Autodesk Inventor part; units mm, degrees
ref_plane "YZ Plane" through (0, 0, 0) normal (1, 0, 0) x (0, 1, 0)
ref_plane "XZ Plane" through (0, 0, 0) normal (0, 1, 0) x (-1, 0, 0)
ref_plane "XY Plane" through (0, 0, 0) normal (0, 0, 1) x (1, 0, 0)
sketch "Эскиз1" plane through (0, 0, 0) normal (0, 1, 0) x (-1, 0, 0)
  line L0 (75.318, 42.5) -> (-75.318, 42.5)
  line L1 (-75.318, 42.5) -> (-75.318, -42.5)
  line L2 (-75.318, -42.5) -> (75.318, -42.5)
  line L3 (75.318, -42.5) -> (75.318, 42.5)
  line L4 (75.318, 42.5) -> (-75.318, -42.5) construction
  line L5 (-75.318, 42.5) -> (75.318, -42.5) construction
  point P0 (0, 0)
  dimension "d0" = 150.636
  dimension "d1" = 85
extrude "Выдавливание1" add sketch "Эскиз1" along normal mid plane 3
sketch "Эскиз3" plane through (-75.318, -1.5, 42.5) normal (-1, 0, 0) x (0, 0, 1)
  line L0 (-85, 0) -> (0, 0)
  line L1 (-80, 3) -> (-70, 3)
  line L2 (-70, 3) -> (-70, 0)
  line L3 (-70, 0) -> (-80, 0)
  line L4 (-80, 0) -> (-80, 3)
  line L5 (-80, 3) -> (-70, 0) construction
  line L6 (-70, 3) -> (-80, 0) construction
  line L7 (-60, 3) -> (-50, 3)
  line L8 (-50, 3) -> (-50, 0)
  line L9 (-50, 0) -> (-60, 0)
  line L10 (-60, 0) -> (-60, 3)
  line L11 (-60, 3) -> (-50, 0) construction
  line L12 (-50, 3) -> (-60, 0) construction
  line L13 (-35, 3) -> (-25, 3)
  line L14 (-25, 3) -> (-25, 0)
  line L15 (-25, 0) -> (-35, 0)
  line L16 (-35, 0) -> (-35, 3)
  line L17 (-35, 3) -> (-25, 0) construction
  line L18 (-25, 3) -> (-35, 0) construction
  line L19 (-15, 3) -> (-5, 3)
  line L20 (-5, 3) -> (-5, 0)
  line L21 (-5, 0) -> (-15, 0)
  line L22 (-15, 0) -> (-15, 3)
  line L23 (-15, 3) -> (-5, 0) construction
  line L24 (-5, 3) -> (-15, 0) construction
  line L25 (0, 0) -> (0, 3)
  line L26 (-85, 0) -> (-85, 3)
  point P0 (-42.5, 1.5)
  point P1 (-75, 1.5)
  point P2 (-55, 1.5)
  point P3 (-30, 1.5)
  point P4 (-10, 1.5)
  point P5 (-15, 1.5)
  point P6 (-25, 1.5)
  point P7 (-60, 1.5)
  point P8 (-35, 0)
  point P9 (-15, 0)
  dimension "d8" = 10
  dimension "d9" = 10
  dimension "d10" = 10
  dimension "d11" = 10
  dimension "d12" = 3
  dimension "d13" = 10
  dimension "d14" = 10
  dimension "d15" = 5
  dimension "d16" = 5
extrude "Выдавливание3" add sketch "Эскиз3" along normal blind 3
sketch "Эскиз4" plane through (75.318, -1.5, -42.5) normal (1, 0, 0) x (0, 0, -1)
  line L0 (-85, 3) -> (0, 3)
  line L1 (-80, 0.0026) -> (-70, 0.0026)
  line L2 (-70, 0.0026) -> (-70, 3)
  line L3 (-70, 3) -> (-80, 3)
  line L4 (-80, 3) -> (-80, 0.0026)
  line L5 (-80, 0.0026) -> (-70, 3) construction
  line L6 (-70, 0.0026) -> (-80, 3) construction
  line L7 (-60, 0.0026) -> (-50, 0.0026)
  line L8 (-50, 0.0026) -> (-50, 3)
  line L9 (-50, 3) -> (-60, 3)
  line L10 (-60, 3) -> (-60, 0.0026)
  line L11 (-60, 0.0026) -> (-50, 3) construction
  line L12 (-50, 0.0026) -> (-60, 3) construction
  line L13 (-42.5, 3) -> (-42.5, 0) construction
  line L14 (0, 0) -> (-85, 0)
  line L15 (-5, 0.0026) -> (-15, 0.0026)
  line L16 (-15, 0.0026) -> (-15, 3)
  line L17 (-15, 3) -> (-5, 3)
  line L18 (-5, 3) -> (-5, 0.0026)
  line L19 (-5, 0.0026) -> (-15, 3) construction
  line L20 (-15, 0.0026) -> (-5, 3) construction
  line L21 (-25, 0.0026) -> (-35, 0.0026)
  line L22 (-35, 0.0026) -> (-35, 3)
  line L23 (-35, 3) -> (-25, 3)
  line L24 (-25, 3) -> (-25, 0.0026)
  line L25 (-25, 0.0026) -> (-35, 3) construction
  line L26 (-35, 0.0026) -> (-25, 3) construction
  line L27 (-85, 3) -> (-85, 0)
  point P0 (-42.5, 1.5)
  point P1 (-75, 1.5013)
  point P2 (-55, 1.5013)
  point P3 (-10, 1.5013)
  point P4 (-30, 1.5013)
  point P5 (-35, 3)
  point P6 (-5, 3)
  point P7 (-15, 3)
  dimension "d19" = 10
  dimension "d24" = 20
  dimension "d29" = 5
extrude "Выдавливание4" add sketch "Эскиз4" along normal blind 3
sketch "Эскиз5" plane through (0, 1.5, 0) normal (0, 1, 0) x (1, 0, 0)
  line L0 (-75.318, 7.5) -> (-75.318, -7.5)
  line L1 (-54.4999, -2.8628) -> (-54.4999, -9.8628)
  line L2 (-54.4999, -9.8628) -> (-48.4999, -9.8628)
  line L3 (-48.4999, -9.8628) -> (-48.4999, -2.8628)
  line L4 (-48.4999, -2.8628) -> (-54.4999, -2.8628)
  line L5 (-48.4999, 3.1372) -> (-48.4999, 10.1372)
  line L6 (-48.4999, 10.1372) -> (-54.4999, 10.1372)
  line L7 (-54.4999, 10.1372) -> (-54.4999, 3.1372)
  line L8 (-54.4999, 3.1372) -> (-48.4999, 3.1372)
  line L9 (-51.4999, -2.8628) -> (-51.4999, 3.1372)
  circle A0 centre (-51.4999, 0.1372) radius 1.5
  point P0 (0, 0)
  dimension "d37" = 3
extrude "Выдавливание5" cut sketch "Эскиз5" against normal blind 3
sketch "Эскиз6" plane through (0, 1.5, 0) normal (0, 1, 0) x (1, 0, 0)
  line L0 (75.318, -27.5) -> (75.318, -17.5)
  line L1 (60.318, -24) -> (60.318, -21)
  line L2 (75.318, -21) -> (75.318, -24)
  line L3 (67.818, -25.55) -> (65.318, -25.55)
  line L4 (65.318, -19.45) -> (67.818, -19.45)
  line L5 (67.818, -19.45) -> (67.818, -21)
  line L6 (67.818, -24) -> (67.818, -25.55)
  line L7 (75.318, -24) -> (67.818, -24)
  line L8 (65.318, -24) -> (60.318, -24)
  line L9 (65.318, -25.55) -> (65.318, -24)
  line L10 (65.318, -21) -> (65.318, -19.45)
  line L11 (60.318, -21) -> (65.318, -21)
  line L12 (67.818, -21) -> (75.318, -21)
  line L13 (66.568, 0) -> (53.2147, 0) construction
  line L14 (0, -10.2584) -> (0, 8.5624) construction
  line L15 (75.318, 27.5) -> (75.318, 17.5)
  line L16 (60.318, 24) -> (60.318, 21)
  line L17 (75.318, 21) -> (75.318, 24)
  line L18 (67.818, 25.55) -> (65.318, 25.55)
  line L19 (65.318, 19.45) -> (67.818, 19.45)
  line L20 (67.818, 19.45) -> (67.818, 21)
  line L21 (67.818, 24) -> (67.818, 25.55)
  line L22 (75.318, 24) -> (67.818, 24)
  line L23 (65.318, 24) -> (60.318, 24)
  line L24 (65.318, 25.55) -> (65.318, 24)
  line L25 (65.318, 21) -> (65.318, 19.45)
  line L26 (60.318, 21) -> (65.318, 21)
  line L27 (67.818, 21) -> (75.318, 21)
  line L28 (0, 10.2584) -> (0, -8.5624) construction
  line L29 (-75.318, -27.5) -> (-75.318, -17.5)
  line L30 (-60.318, -24) -> (-60.318, -21)
  line L31 (-75.318, -21) -> (-75.318, -24)
  line L32 (-67.818, -25.55) -> (-65.318, -25.55)
  line L33 (-65.318, -19.45) -> (-67.818, -19.45)
  line L34 (-67.818, -19.45) -> (-67.818, -21)
  line L35 (-67.818, -24) -> (-67.818, -25.55)
  line L36 (-75.318, -24) -> (-67.818, -24)
  line L37 (-65.318, -24) -> (-60.318, -24)
  line L38 (-65.318, -25.55) -> (-65.318, -24)
  line L39 (-65.318, -21) -> (-65.318, -19.45)
  line L40 (-60.318, -21) -> (-65.318, -21)
  line L41 (-67.818, -21) -> (-75.318, -21)
  line L42 (-66.568, 0) -> (-53.2147, 0) construction
  line L43 (-60.318, 24) -> (-60.318, 21)
  line L44 (-65.318, 24) -> (-60.318, 24)
  line L45 (-60.318, 21) -> (-65.318, 21)
  line L46 (-65.318, 21) -> (-65.318, 19.45)
  line L47 (-65.318, 19.45) -> (-67.818, 19.45)
  line L48 (-67.818, 19.45) -> (-67.818, 21)
  line L49 (-65.318, 25.55) -> (-65.318, 24)
  line L50 (-67.818, 25.55) -> (-65.318, 25.55)
  line L51 (-67.818, 24) -> (-67.818, 25.55)
  line L52 (-67.818, 21) -> (-75.318, 21)
  line L53 (-75.318, 21) -> (-75.318, 24)
  line L54 (-75.318, 27.5) -> (-75.318, 17.5)
  line L55 (-75.318, 24) -> (-67.818, 24)
  point P0 (0, 0)
  point P1 (67.818, -23.3834)
  point P2 (67.818, 23.3834)
  point P3 (-67.818, -23.3834)
  point P4 (-67.818, 23.3834)
  point P5 (-75.318, -21)
  point P6 (75.318, -22.5)
  dimension "d38" = 6.1
  dimension "d39" = 3
  dimension "d40" = 2.5
  dimension "d41" = 15
  dimension "d42" = 1.55
  dimension "d43" = 1.55
  dimension "d44" = 1.55
  dimension "d45" = 1.55
extrude "Выдавливание6" cut sketch "Эскиз6" against normal blind 3
properties part number "Нижняя часть головы"
Here's how the part is built. I have some questions about the finished solid (model axes, mm). A direction names the side the tool comes from. Give positions to 0.01 mm unless a question says otherwise; leave off trailing zeros. Loops run counter-clockwise (first coordinate to the right, second up) from the corner with the lowest first, then second, coordinate; pieces in that order, holes last. Notation, with made-up numbers: (-2, 24.25) -> (26, 24.25) arc R15 ccw to (26, 47.25) -> close; hole circle Ø9 at (-21.75, 70). An arc over 180 degrees is marked (long way). Answer as a JSON object with one key per item and string values. Group by question number.
Item 1: I need wall thicknesses on L1, parallel to Z at x = 68, y = -0.25; L2, parallel to X at y = 0.3, z = -25.5; L3, parallel to Z at x = -67, y = 0.75. Which ranges of each line are inside material? Lowest first, please.
Item 2: Imagine slicing it at B-B on y = 0.05. Give the number of separate pieces and of enclosed holes in the cut face, then the cut area to 3 significant figures.
Item 3: On a 3-axis mill with a long thin cutter (end or side, diameter ignored), from which of +Z, -Z, +X, -X, +Y, -Y can I reach the whole of each face in a straight line? I mean faces 1 (the flat face through (-75.318, 0, -40)), 2 (the flat face through (-63, 0, 24)), 3 (the flat face through (60.318, 0, -23)). Say none if no direction works.
Item 4: Thinking about a two-plate mould opening in Z: for faces 4 (the flat face through (63, 0, -24)), 5 (the flat face through (77, -1.497, 33)), which applies, pulls with the +Z half, pulls with the -Z half, needs draft (parallel to the pull), parting line crosses it, or undercut?
Item 5: Will these pins go through, and if not, where does the flat tip stop? pin 1 (0.8 mm diameter, centred on y = -0.5, z = 24.5, fed in from -X); pin 2 (0.5 mm diameter, centred on y = 0.5, z = 25, fed in from +X); pin 3 (1.5 mm diameter, centred on x = -77, y = 0.5, fed in from +Z).
Item 6: Imagine slicing it at A-A on z = 5. Write out the boundary of the cut face in (x, y), then the cut area to 3 significant figures.
Answer list:
{
 "1": {"L1": "z = -42.5 to -24, -21 to 21, 24 to 42.5", "L2": "x = -75.32 to -67.82, -65.32 to 65.32, 67.82 to 75.32", "L3": "z = -42.5 to -25.55, -19.45 to 19.45, 25.55 to 42.5"},
 "2": {"separate pieces": "1", "enclosed holes": "3", "area": "12,700 mm2"},
 "3": {"face 1": "-Z, -X, +Y, -Y", "face 2": "-X, +Y, -Y", "face 3": "+X, +Y, -Y"},
 "4": {"face 4": "undercut", "face 5": "needs draft"},
 "5": {"pin 1": "stops at x = -75.32", "pin 2": "stops at x = 75.32", "pin 3": "stops at z = 37.5"},
 "6": {"outline": "(-75.32, -1.5) -> (-54.5, -1.5) -> (-54.5, 1.5) -> (-75.32, 1.5) -> close; (-48.5, -1.5) -> (75.32, -1.5) -> (75.32, 1.5) -> (-48.5, 1.5) -> close", "area": "434 mm2"}
}
